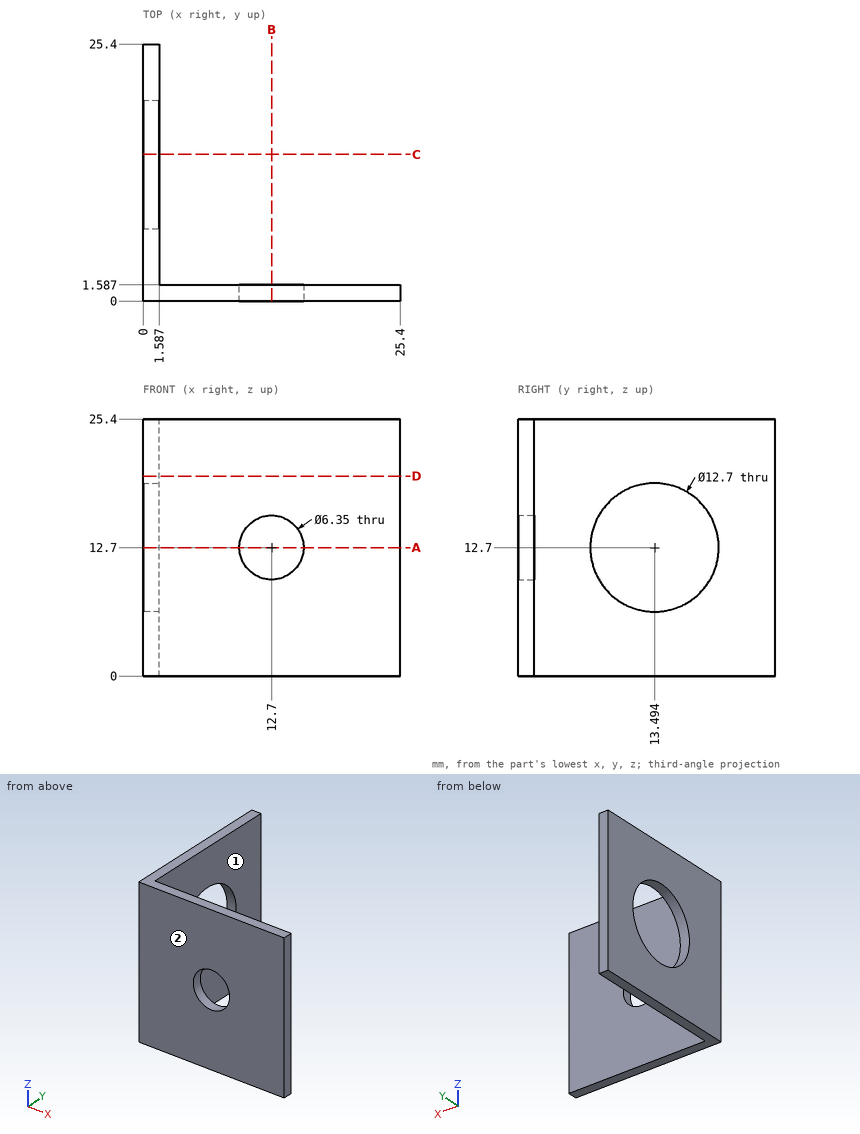
Geometry: see drawing. Coordinates: mm, zero at the bounding-box minimum. A direction names the side the tool comes from. Give positions to 0.01 mm unless a question says otherwise; leave off trailing zeros. Order: outer loops, then holes, each group sorted by start corner. A loop starts at its lowest first (then second) coordinate and runs counter-clockwise, first axis right, second up. Notation, with made-up numbers: (-13, 35) - (44, 35) arc R32 ccw to (44, 73) - close; hole circle Ø4 at (16.25, 70). An arc over 180 degrees is marked (long way). Use a Markdown table: item, result.
(1) Section query A-A (z = 12.7). Output: boundary loops of the cut face in (x, y) (1 decimal).
Computed values:
| item | result |
|---|---|
| outline | (0, 0) - (9.5, 0) - (9.5, 1.6) - (1.6, 1.6) - (1.6, 7.1) - (0, 7.1) - close; (0, 19.8) - (1.6, 19.8) - (1.6, 25.4) - (0, 25.4) - close; (15.9, 0) - (25.4, 0) - (25.4, 1.6) - (15.9, 1.6) - close |
(2) Section query D-D (z = 19.75). Output: boundary loops of the cut face in (x, y).
Computed values:
| item | result |
|---|---|
| outline | (0, 0) - (25.4, 0) - (25.4, 1.59) - (1.59, 1.59) - (1.59, 25.4) - (0, 25.4) - close |
(3) Access query for the marked faces 1 and 2. Directions: +Z, -Z, +X, -X, +Y, -Y. A direction counts if a zero-diameter tool reaches every point of the face in a straight line with its end or side. Return the directions, or none.
Computed values:
| item | result |
|---|---|
| face 1 | +Z, -Z, +X, +Y |
| face 2 | +Z, -Z, +X, -X, -Y |
(4) Section query C-C (y = 14.5). Output: boundary loops of the cut face in (x, z).
Computed values:
| item | result |
|---|---|
| outline | (0, 0) - (1.59, 0) - (1.59, 6.43) - (0, 6.43) - close; (0, 18.97) - (1.59, 18.97) - (1.59, 25.4) - (0, 25.4) - close |
(5) Section query B-B (x = 12.7). Output: boundary loops of the cut face in (y, z) (1 decimal).
Computed values:
| item | result |
|---|---|
| outline | (0, 0) - (1.6, 0) - (1.6, 9.5) - (0, 9.5) - close; (0, 15.9) - (1.6, 15.9) - (1.6, 25.4) - (0, 25.4) - close |
(6) Pin query (flat end, axial travel): pin 1 (8.5 mm diameter, centred on x = 12.7, z = 12.7, fed in from +Y); pin 2 (10 mm diameter, centred on y = 4.5, z = 22, fed in from -X); pin 3 (5 mm diameter, centred on x = 5.5, y = 9.5, fed in from -Z). Return the tip coordinate at first contact, or that it passes through.
Computed values:
| item | result |
|---|---|
| pin 1 | stops at y = 1.59 |
| pin 2 | stops at x = 0 |
| pin 3 | passes through |
(7) Line query: line 1 (X direction, y = 0.6, z = 12.7) (1 decimal); line 2 (Y direction, x = 0.4, z = 12.7). Output: solid intervals per line, ascending. Write a range as from..to.
Computed values:
| item | result |
|---|---|
| line 1 | x = 0..9.5, 15.9..25.4 |
| line 2 | y = 0..7.14, 19.84..25.4 |
